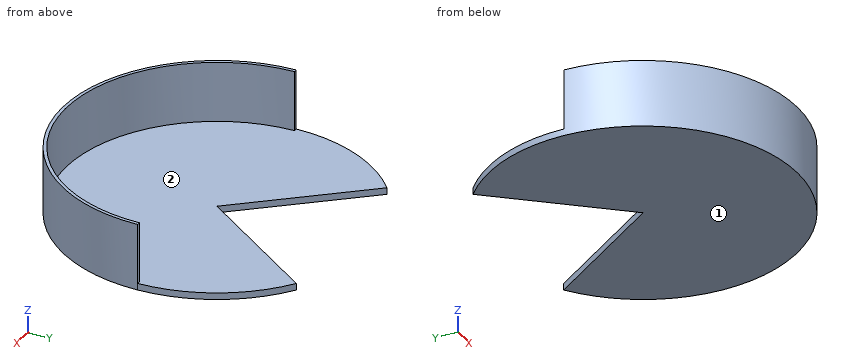
from build123d import *

# Parameters (mm, degrees)
F0_R     = 146.05
F1_DEPTH = 63.5
F2_R     = 142.875
F3_DEPTH = 57.15
F5_DEPTH = 57.15
F7_DEPTH = 63.501


with BuildPart() as f1:
    # F0 (on Top) → F1 (new body)
    with BuildSketch(Plane.XY):
        Circle(F0_R)
    extrude(amount=F1_DEPTH)

    # F2 (on face) → F3 (cut)
    with BuildSketch(Plane.XY.offset(63.5)):
        Circle(F2_R)
    extrude(amount=-F3_DEPTH, mode=Mode.SUBTRACT)

    # F4 (on face) → F5 (cut)
    with BuildSketch(Plane.XY.offset(63.5)):
        with BuildLine():
            Line((142.875, 0), (186.450183, 0))
            Line((186.450183, 0), (186.450183, 147.836223))
            Line((186.450183, 147.836223), (-190.863192, 147.836223))
            Line((-190.863192, 147.836223), (-190.863192, 0))
            Line((-190.863192, 0), (-142.875, 0))
            ThreePointArc((-142.875, 0), (0, 142.875), (142.875, 0))
        make_face()
    extrude(amount=-F5_DEPTH, mode=Mode.SUBTRACT)

    # F6 (on face) → F7 (cut, through all)
    with BuildSketch(Plane.XY.offset(63.5)):
        with BuildLine():
            Line((0, 0), (92.831509, 128.778389))
            ThreePointArc((92.831509, 128.778389), (-4.756055, 152.325769), (-100.68453, 122.736254))
            Line((-100.68453, 122.736254), (0, 0))
        make_face()
    extrude(amount=-F7_DEPTH, mode=Mode.SUBTRACT)


solid = f1.part
CAD build for the part. Positions are in the model's coordinates, mm. Face numbers are marked on the shaded views. Coordinates: 2 decimals unless noted, no trailing zeros. Write each loop counter-clockwise with the first axis right and the second up, starting at its lowest first coordinate (ties: lowest second). Pieces come first, ordered by that corner, then holes. Notation, with made-up numbers: M 89,-1 L 95,-1 A5 cw 95,4 Z; hole C 62.5,74.25 d7. An arc over 180 degrees is marked long. Answer as a JSON object with one key per item and string values. Group by question number.
1) Wall check: line 1 (Z direction, x = 110, y = 25.5); line 2 (X direction, y = -110, z = 16.5); line 3 (X direction, y = -17.5, z = 13.5). Give the ranges that are in metal, low to high. Write a range as from..to.
2) Pin check, flat tips, straight feed: pin 1 Ø5 at (x, z) = (10, 6.5) entering from +Y; pin 2 Ø3 at (x, y) = (-46, 24.5) entering from +Z; pin 3 Ø6 at (x, z) = (66.5, 38) entering from -Y. Stop position of each tip, or through.
3) Saw through at A-A (y = 93). Write the cut outline in (x, z).
4) Mould opens along X. For the marked faces 1 and 2 say: +X half, -X half, draft (parallel to the pull), parting line (faces both ways), or undercut.
5) Saw through at D-D (y = 60). Write the cut outline in (x, z), plus the area to 3 significant figures.
6) Saw through at B-B (z = 56). Write the cut outline in (x, y) (3 decimals).
7) Saw through at C-C (x = 116). Write the cut outline in (y, z).
Values follow:
{
 "1": {"line 1": "z = 0..6.35", "line 2": "x = -96.08..-91.18, 91.18..96.08", "line 3": "x = -145..-141.8, 141.8..145"},
 "2": {"pin 1": "stops at y = 17.33", "pin 2": "stops at z = 6.35", "pin 3": "stops at y = -131.52"},
 "3": {"outline": "M -112.61,0 L -76.29,0 L -76.29,6.35 L -112.61,6.35 Z; M 67.04,0 L 112.61,0 L 112.61,6.35 L 67.04,6.35 Z"},
 "4": {"face 1": "draft", "face 2": "undercut"},
 "5": {"outline": "M -133.16,0 L -49.22,0 L -49.22,6.35 L -133.16,6.35 Z; M 43.25,0 L 133.16,0 L 133.16,6.35 L 43.25,6.35 Z", "area": "1,100 mm2"},
 "6": {"outline": "M -146.05,0 A146.05 ccw 146.05,0 L 142.875,0 A142.875 cw -142.875,0 Z"},
 "7": {"outline": "M -88.74,0 L 88.74,0 L 88.74,6.35 L -83.41,6.35 L -83.41,63.5 L -88.74,63.5 Z"}
}
